The model under review builds one solid part; all positions refer to its coordinate system, in mm. A direction names the side the tool comes from. Give positions to 0.01 mm unless a question says otherwise; leave off trailing zeros. Loops run counter-clockwise (first coordinate to the right, second up) from the corner with the lowest first, then second, coordinate; pieces in that order, holes last. Notation, with made-up numbers: M 13,-8 L 67,-8 A20 cw 67,30 Z; hole C -22,17 d3. An arc over 180 degrees is marked long. Return JSON: item names as keys, results as strings.
```python
from build123d import *

# Parameters (mm, degrees)
SKETCH1_R           = 3.75
SKETCH1_R_2         = 1.375
BOSS_EXTRUDE1_DEPTH = 6.35


with BuildPart() as part:
    # Sketch1 → Boss-Extrude1 (new body)
    with BuildSketch(Plane(origin=(0, 0, 0), x_dir=(-1, 0, 0), z_dir=(0, 0, -1))):
        with BuildLine():
            Line((-106.79268786, -4.343029528), (-107.882772007, -4.343029528))
            ThreePointArc((-107.882772007, -4.343029528), (-104.997693278, -7.484855503), (-100.99, -8.945384285))
            Line((-100.99, -8.945384285), (-2.2, -19.878631744))
            ThreePointArc((-2.2, -19.878631744), (4.756528256, -19.426153478), (11.135161851, -16.613493629))
            ThreePointArc((11.135161851, -16.613493629), (11.586893238, -16.409333237), (12.080499812, -16.363559202))
            ThreePointArc((12.080499812, -16.363559202), (15.202795796, -15.202795795), (16.363559202, -12.080499812))
            ThreePointArc((16.363559202, -12.080499812), (16.409333237, -11.586893238), (16.613493629, -11.135161851))
            ThreePointArc((16.613493629, -11.135161851), (20, 0), (16.613493629, 11.135161851))
            ThreePointArc((16.613493629, 11.135161851), (16.409333237, 11.586893238), (16.363559202, 12.080499812))
            ThreePointArc((16.363559202, 12.080499812), (15.202795795, 15.202795795), (12.080499812, 16.363559202))
            ThreePointArc((12.080499812, 16.363559202), (11.586893238, 16.409333237), (11.135161851, 16.613493629))
            ThreePointArc((11.135161851, 16.613493629), (4.756528256, 19.426153478), (-2.2, 19.878631744))
            Line((-2.2, 19.878631744), (-100.99, 8.945384285))
            ThreePointArc((-100.99, 8.945384285), (-104.997693278, 7.484855504), (-107.882772007, 4.343029529))
            Line((-107.882772007, 4.343029529), (-106.79268786, 4.343029529))
            Line((-106.79268786, 4.343029529), (-106.79268786, -4.343029528))
        make_face()
        with Locations((-100, 0)):
            Circle(SKETCH1_R, mode=Mode.SUBTRACT)
        with Locations((12.374368671, -12.374368671)):
            Circle(SKETCH1_R_2, mode=Mode.SUBTRACT)
        with Locations((12.374368671, 12.374368671)):
            Circle(SKETCH1_R_2, mode=Mode.SUBTRACT)
        with Locations((-12.374368671, 12.374368671)):
            Circle(SKETCH1_R_2, mode=Mode.SUBTRACT)
        with Locations((-12.374368671, -12.374368671)):
            Circle(SKETCH1_R_2, mode=Mode.SUBTRACT)
        with BuildLine():
            Line((-18.281656562, -13.06832175), (-90.303846884, -5.097510642))
            ThreePointArc((-90.303846884, -5.097510642), (-91.413718881, -4.396993797), (-91.547583043, -3.091382795))
            ThreePointArc((-91.547583043, -3.091382795), (-91, 0), (-91.547583043, 3.091382796))
            ThreePointArc((-91.547583043, 3.091382796), (-91.413718881, 4.396993797), (-90.303846884, 5.097510642))
            Line((-90.303846884, 5.097510642), (-18.281656562, 13.068321749))
            ThreePointArc((-18.281656562, 13.068321749), (-16.842747955, 12.369356727), (-16.852703779, 10.769697087))
            ThreePointArc((-16.852703779, 10.769697087), (-20, 0), (-16.852703779, -10.769697087))
            ThreePointArc((-16.852703779, -10.769697087), (-16.842747955, -12.369356727), (-18.281656562, -13.06832175))
        make_face(mode=Mode.SUBTRACT)
        with BuildLine():
            ThreePointArc((-11.80010118, -8.415806198), (-12.416598495, -8.179555802), (-12.871945412, -7.701494746))
            ThreePointArc((-12.871945412, -7.701494746), (-15, 0), (-12.871945412, 7.701494746))
            ThreePointArc((-12.871945412, 7.701494746), (-12.416598495, 8.179555802), (-11.80010118, 8.415806198))
            ThreePointArc((-11.80010118, 8.415806198), (-9.545941546, 9.545941546), (-8.415806198, 11.80010118))
            ThreePointArc((-8.415806198, 11.80010118), (-8.179555802, 12.416598495), (-7.701494746, 12.871945412))
            ThreePointArc((-7.701494746, 12.871945412), (0, 15), (7.701494746, 12.871945412))
            ThreePointArc((7.701494746, 12.871945412), (8.179555802, 12.416598495), (8.415806198, 11.80010118))
            ThreePointArc((8.415806198, 11.80010118), (9.545941546, 9.545941546), (11.80010118, 8.415806198))
            ThreePointArc((11.80010118, 8.415806198), (12.416598495, 8.179555802), (12.871945412, 7.701494746))
            ThreePointArc((12.871945412, 7.701494746), (15, 0), (12.871945412, -7.701494746))
            ThreePointArc((12.871945412, -7.701494746), (12.416598495, -8.179555803), (11.80010118, -8.415806198))
            ThreePointArc((11.80010118, -8.415806198), (9.545941546, -9.545941546), (8.415806198, -11.80010118))
            ThreePointArc((8.415806198, -11.80010118), (8.179555803, -12.416598495), (7.701494746, -12.871945412))
            ThreePointArc((7.701494746, -12.871945412), (0, -15), (-7.701494746, -12.871945412))
            ThreePointArc((-7.701494746, -12.871945412), (-8.179555802, -12.416598495), (-8.415806198, -11.80010118))
            ThreePointArc((-8.415806198, -11.80010118), (-9.545941546, -9.545941546), (-11.80010118, -8.415806198))
        make_face(mode=Mode.SUBTRACT)
    extrude(amount=-BOSS_EXTRUDE1_DEPTH)


solid = part.part
```
1) Insertion check: pin 1 (4.5 mm diameter, centred on x = 12.37, y = -12.37, fed in from -Z); pin 2 (0.9 mm diameter, centred on x = 107.5, z = 2.5, fed in from +Y); pin 3 (1 mm diameter, centred on x = 87, z = 4.5, fed in from +Y). Each pin has a flat end and moves straight along its axis. Give the tip position at first contact, or say it passes through.
From the geometry:
{"pin 1": "z = 0", "pin 2": "y = 5.59", "pin 3": "y = 10.55"}
2) Consider section D-D on z = 1. Count the separate pieces of the cut face and the enclosed holes in it, then the cut area to 3 significant figures.
From the geometry:
{"separate pieces": "1", "enclosed holes": "7", "area": "1,610 mm²"}
3) Wall thickness on L1, parallel to Y at x = 12, z = 5.25; L2, parallel to X at y = -2.5, z = 6.25; L3, parallel to X at y = 1, z = 1.25: over which ranges is each line inside the solid? List them lowest first. Write a range as from..to.
From the geometry:
{"L1": "-18.79..-13.7, -11.05..-8.37, 8.37..11.05, 13.7..18.79", "L2": "-19.84..-14.79, 14.79..19.84, 91.35..97.2, 102.8..106.79", "L3": "-19.97..-14.97, 14.97..19.97, 91.06..96.39, 103.61..106.79"}
4) Consider section A-A on y = 0. Write out the cut boundary in (x, z).
From the geometry:
{"outline": "M -20,0 L -15,0 L -15,6.35 L -20,6.35 Z; M 15,0 L 20,0 L 20,6.35 L 15,6.35 Z; M 91,0 L 96.25,0 L 96.25,6.35 L 91,6.35 Z; M 103.75,0 L 106.79,0 L 106.79,6.35 L 103.75,6.35 Z"}
5) Consider section B-B on y = -6.5. Write out the cut boundary in (x, z), then the cut area to 3 significant figures.
From the geometry:
{"outline": "M -18.91,0 L -13.52,0 L -13.52,6.35 L -18.91,6.35 Z; M 13.52,0 L 18.91,0 L 18.91,6.35 L 13.52,6.35 Z; M 77.63,0 L 106.22,0 L 106.22,6.35 L 77.63,6.35 Z", "area": "250 mm²"}
6) Tool access review of faces 4 (the face through (9.52, -9.57, 3.13)), 5 (the face through (105.05, -7.45, 3.13)): name each direction out of +Z, -Z, +X, -X, +Y, -Y from which nothing blocks a thin tool from reaching the whole face with its end or side.
From the geometry:
{"face 4": "+Z, -Z", "face 5": "+Z, -Z, +X, -Y"}
7) The part is to be moulded in two halves that separate along X. For faces 1 (the face through (-20, 0, 3)), 2 (the face through (106.793, 0, 3)), 3 (the face through (12.67, 11.03, 3.13)), say which applies: released by +X, released by -X, zero draft, split by the parting line, or undercut.
From the geometry:
{"face 1": "released by -X", "face 2": "released by +X", "face 3": "undercut"}
8) Consider section C-C on x = 29. Write out the cut boundary in (y, z), then the cut area to 3 significant figures.
From the geometry:
{"outline": "M -16.91,0 L -11.88,0 L -11.88,6.35 L -16.91,6.35 Z; M 11.88,0 L 16.91,0 L 16.91,6.35 L 11.88,6.35 Z", "area": "63.9 mm²"}
